Check sheet for the drawn part. Datum: minimum x, y, z corner. Units: mm. Coordinates: 2 decimals unless noted, no trailing zeros. Order: outer loops, then holes, each group sorted by start corner. A loop starts at its lowest first (then second) coordinate and runs counter-clockwise, first axis right, second up.
1. Thickness scan on line 1 (Z direction, x = 22, y = 19); line 2 (Z direction, x = 26, y = 4); line 3 (Z direction, x = 26, y = 18). Record the ranges inside material, lowest first.
2. Cross-section at A-A (x = 20). Enter the section's corners in (y, z), then the cut area to 3 significant figures.
3. Draft check along Y on the marked faces 1 and 2. Enter one of: released by +Y, released by -Y, zero draft, split by the parting line, or undercut.
4. Cross-section at D-D (y = 8.5). Enter the section's corners in (x, z).
5. Cross-section at B-B (x = 7). Enter the section's corners in (y, z).
6. Gauge pin test, flat ends, axial feed: pin 1 Ø3 at (x, z) = (30, 30.5) entering from -Y; pin 2 Ø5 at (y, z) = (19, 85) entering from -X; pin 3 Ø3 at (y, z) = (27, 43) entering from +X. Record the tip position at first contact, or that the pin passes through.
7. Cross-section at C-C (z = 61). Enter the section's corners in (x, y), then the cut area to 3 significant figures.
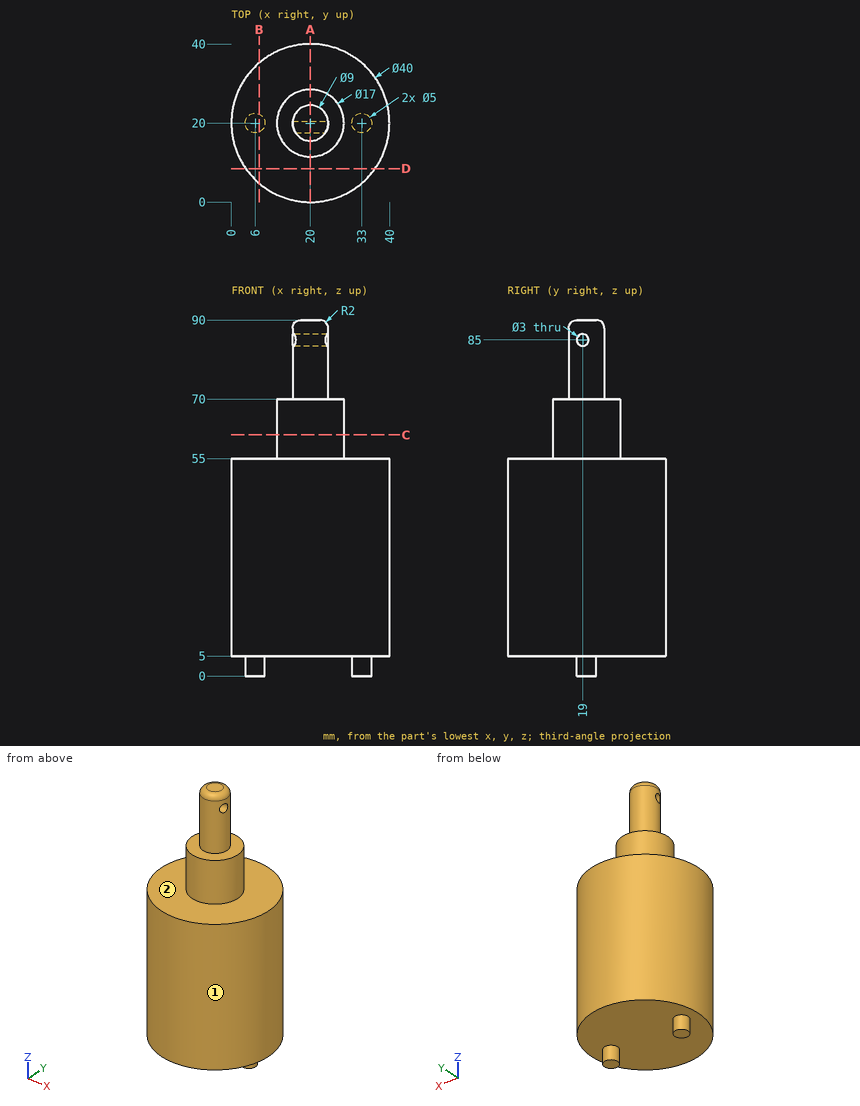
Data:
1. line 1: z = 5 to 83.5, 86.5 to 90
1. line 2: z = 5 to 55
1. line 3: z = 5 to 70
2. outline: (0, 5) - (40, 5) - (40, 55) - (28.5, 55) - (28.5, 70) - (24.5, 70) - (24.5, 88) arc R2 ccw to (22.5, 90) - (17.5, 90) arc R2 ccw to (15.5, 88) - (15.5, 70) - (11.5, 70) - (11.5, 55) - (0, 55) - close; hole circle Ø3 at (19, 85)
2. area: 2,430 mm2
3. face 1: split by the parting line
3. face 2: zero draft
4. outline: (3.64, 5) - (36.36, 5) - (36.36, 55) - (3.64, 55) - close
5. outline: (4.8, 5) - (17.71, 5) - (17.71, 0) - (22.29, 0) - (22.29, 5) - (35.2, 5) - (35.2, 55) - (4.8, 55) - close
6. pin 1: stops at y = 1.9
6. pin 2: stops at x = 15.5
6. pin 3: stops at x = 39.23
7. outline: circle Ø17 at (20, 20)
7. area: 227 mm2
